```python
from build123d import *

# Parameters (mm, degrees)
SKETCH_1_W               = 160
SKETCH_1_H               = 60
EXTRUDE_1_DEPTH          = 30
SKETCH_2_W               = 20
SKETCH_2_H               = 40
CUT_EXTRUDE_1_DEPTH      = 171
SKETCH_3_W               = 95
SKETCH_3_H               = 90
CUT_EXTRUDE_2_DEPTH      = 171
FILLET_1_R               = 5
EXTRUDE_2_DEPTH          = 5
EXTRUDE_START            = 5
EXTRUDE_3_DEPTH          = 5
CUT_EXTRUDE_3_DEPTH      = 91
CUT_EXTRUDE_3_DEPTH_BACK = 33
SKETCH_6_R               = 4


with BuildPart() as part:
    # 草图1 → 凸台-拉伸1 (new body)
    with BuildSketch(Plane.XY):
        Rectangle(SKETCH_1_W, SKETCH_1_H)
    extrude(amount=EXTRUDE_1_DEPTH)

    # 草图2 → 切除-拉伸1 (cut)
    with BuildSketch(Plane.ZY.offset(80)):
        with Locations((15, -30)):
            Rectangle(SKETCH_2_W, SKETCH_2_H)
    extrude(amount=-CUT_EXTRUDE_1_DEPTH, mode=Mode.SUBTRACT)

    # 草图3 → 切除-拉伸2 (cut)
    with BuildSketch(Plane.XY.offset(30)):
        with Locations((0, -30)):
            Rectangle(SKETCH_3_W, SKETCH_3_H)
    extrude(amount=-CUT_EXTRUDE_2_DEPTH, mode=Mode.SUBTRACT)

    # 圆角1
    fillet_1_edges = [part.edges().sort_by_distance(p)[0] for p in [
        (-47.5, 15, 15),
        (47.5, 15, 15),
    ]]
    fillet(fillet_1_edges, radius=FILLET_1_R)

    # 草图4 → 凸台-拉伸2 (add)
    with BuildSketch(Plane.XY.offset(30)):
        with BuildLine():
            Line((-47.5, -30), (-47.5, 10))
            ThreePointArc((-47.5, 10), (-46.035533906, 13.535533906), (-42.5, 15))
            Line((-42.5, 15), (42.5, 15))
            ThreePointArc((42.5, 15), (46.035533906, 13.535533906), (47.5, 10))
            Line((47.5, 10), (47.5, -30))
            Line((47.5, -30), (80, -30))
            Line((80, -30), (80, 30))
            Line((80, 30), (-80, 30))
            Line((-80, 30), (-80, -30))
            Line((-80, -30), (-47.5, -30))
        make_face()
    extrude(amount=EXTRUDE_2_DEPTH)

    # 草图5 → 凸台-拉伸3 (add)
    with BuildSketch(Plane(origin=(0, 0, 0), x_dir=(-1, 0, 0), z_dir=(0, 0, -1)).offset(EXTRUDE_START)):
        with BuildLine():
            Line((-47.5, -30), (-47.5, 10))
            ThreePointArc((-47.5, 10), (-46.035533906, 13.535533906), (-42.5, 15))
            Line((-42.5, 15), (42.5, 15))
            ThreePointArc((42.5, 15), (46.035533906, 13.535533906), (47.5, 10))
            Line((47.5, 10), (47.5, -30))
            Line((47.5, -30), (80, -30))
            Line((80, -30), (80, 30))
            Line((80, 30), (-80, 30))
            Line((-80, 30), (-80, -30))
            Line((-80, -30), (-47.5, -30))
        make_face()
    extrude(amount=-EXTRUDE_3_DEPTH)

    # 草图6 → 切除-拉伸3 (cut, two sides: drawn at the far end of the back side and taken through both)
    with BuildSketch(Plane.XZ.offset(-15).offset(-CUT_EXTRUDE_3_DEPTH_BACK)):
        with Locations((-63.75, 35)):
            Circle(SKETCH_6_R)
        with Locations((-63.75, -5)):
            Circle(SKETCH_6_R)
        with Locations((63.75, -5)):
            Circle(SKETCH_6_R)
        with Locations((63.75, 35)):
            Circle(SKETCH_6_R)
    extrude(amount=CUT_EXTRUDE_3_DEPTH + CUT_EXTRUDE_3_DEPTH_BACK, mode=Mode.SUBTRACT)


solid = part.part
```
Verification items for the finished model (mm, model axes). A direction names the side the tool comes from. Coordinates: 2 decimals unless noted, no trailing zeros. Loops run counter-clockwise (first coordinate to the right, second up) from the corner with the lowest first, then second, coordinate; pieces in that order, holes last. Notation, with made-up numbers: (58.5, 24) - (92.5, 24) arc R21 ccw to (92.5, 42) - close; hole circle Ø8 at (85, 38.25). An arc over 180 degrees is marked (long way). Return JSON: item names as keys, results as strings.
1. Go/stop test with a flat-tipped pin: pin 1 (6 mm diameter, centred on x = 61, z = 19, fed in from -Y). Record where the tip stops, or that it passes through.
Established:
{"pin 1": "stops at y = -10"}
2. Section check C-C, the plane z = 27.5. Record the boundary of the cut face in (x, y).
Established:
{"outline": "(-80, -30) - (-47.5, -30) - (-47.5, 10) arc R5 cw to (-42.5, 15) - (42.5, 15) arc R5 cw to (47.5, 10) - (47.5, -30) - (80, -30) - (80, 30) - (-80, 30) - close"}
3. Section check D-D, the plane x = 50. Record the boundary of the cut face in (y, z).
Established:
{"outline": "(-30, -5) - (30, -5) - (30, 35) - (-30, 35) - (-30, 25) - (-10, 25) - (-10, 5) - (-30, 5) - close"}
4. Tool access check on faces 1 (the flat face through (47.5, -6, 15)), 2 (the flat face through (64, -20, 5)), 3 (the flat face through (64, -30, 0)). Record the directions out of +Z, -Z, +X, -X, +Y, -Y that give a thin tool (end or side, any length) a straight path to the whole face; none if there is none.
Established:
{"face 1": "+Z, -Z, -Y", "face 2": "+X, -X, -Y", "face 3": "+Z, -Z, +X, -X, -Y"}
5. Thickness scan on L1, parallel to X at y = 5, z = 20; L2, parallel to X at y = 13, z = -2; L3, parallel to Y at x = 11.5, z = 19.5. Record the ranges inside material, lowest first.
Established:
{"L1": "x = -80 to -47.5, 47.5 to 80", "L2": "x = -80 to -66.4, -61.1 to -46.5, 46.5 to 61.1, 66.4 to 80", "L3": "y = 15 to 30"}
6. Mould release check, pull along Z, two halves, no side actions. Record for faces 4 (the flat face through (-64, -30, 30)), 5 (the cylindrical face through (-63.8, 0.4, 31)), 6 (the flat face through (64, -20, 25)), 7 (the cylindrical face through (-63.7, 0.4, -1)): +Z half, -Z half, draft (parallel to the pull), parting line (faces both ways), or undercut.
Established:
{"face 4": "draft", "face 5": "+Z half", "face 6": "undercut", "face 7": "-Z half"}
7. Section check B-B, the plane x = -63.75. Record the boundary of the cut face in (y, z).
Established:
{"outline": "(-30, -1) - (30, -1) - (30, 31) - (-30, 31) - (-30, 25) - (-10, 25) - (-10, 5) - (-30, 5) - close"}
8. Section check A-A, the plane z = 21. Record the boundary of the cut face in (x, y).
Established:
{"outline": "(-80, -10) - (-47.5, -10) - (-47.5, 10) arc R5 cw to (-42.5, 15) - (42.5, 15) arc R5 cw to (47.5, 10) - (47.5, -10) - (80, -10) - (80, 30) - (-80, 30) - close"}
